Geometry: final body of the model. Coordinates: model frame, mm. Give positions to 0.01 mm unless a question says otherwise; leave off trailing zeros. Order: outer loops, then holes, each group sorted by start corner. A loop starts at its lowest first (then second) coordinate and runs counter-clockwise, first axis right, second up. Notation, with made-up numbers: M -18,19.5 L 21,19.5 A21 ccw 21,36.5 Z; hole C -39.75,86 d11. An arc over 180 degrees is marked long. Write item = value, one per line. Start each with the question number.
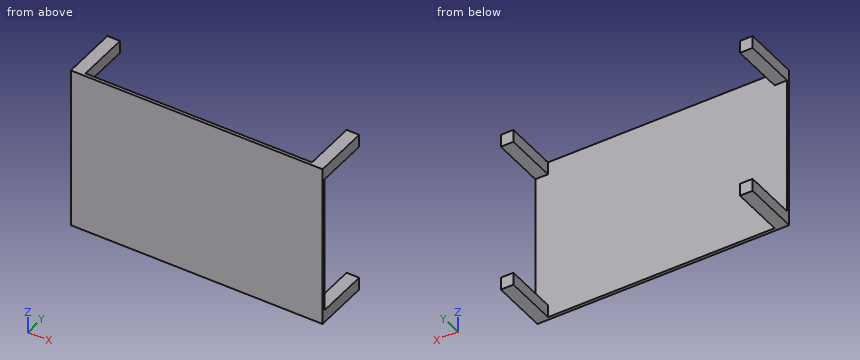
from build123d import *

# Parameters (mm, degrees)
SKETCH2_W            = 254
SKETCH2_H            = 165.1
BOSS_EXTRUDE1_DEPTH  = 3.175
SKETCH3_W            = 12.7
SKETCH3_H            = 12.7
BOSS_EXTRUDE2_DEPTH  = 53.975
LPATTERN1_COUNT      = 2
LPATTERN1_PITCH      = 152.4
LPATTERN1_COUNT_DIR2 = 2
LPATTERN1_PITCH_DIR2 = 241.3


with BuildPart() as part:
    # Sketch2 → Boss-Extrude1 (new body)
    with BuildSketch(Plane(origin=(0, 0, 0), x_dir=(1, 0, 0), z_dir=(0, 1, 0))):
        Rectangle(SKETCH2_W, SKETCH2_H)
    extrude(amount=BOSS_EXTRUDE1_DEPTH)

    # Sketch3 → Boss-Extrude2 (add)
    with BuildSketch(Plane(origin=(0, 3.175, 0), x_dir=(1, 0, 0), z_dir=(0, 1, 0))):
        with Locations((-120.65, -76.2)):
            Rectangle(SKETCH3_W, SKETCH3_H)
    boss_extrude2 = extrude(amount=BOSS_EXTRUDE2_DEPTH)

    # LPattern1: Boss-Extrude2 2 × 2
    with Locations(*[(j * LPATTERN1_PITCH_DIR2, 0, -i * LPATTERN1_PITCH) for i in range(LPATTERN1_COUNT) for j in range(LPATTERN1_COUNT_DIR2) if (i, j) != (0, 0)]):
        add(boss_extrude2)


solid = part.part
1) Cut plane C-C (z = -1). Return loops of the section in (x, y) (3 decimals), plus the area to 3 significant figures.
2) Cut plane A-A (y = 50.5). Return loops of the section in (x, z), plus the area to 3 significant figures.
3) Ray query, L1, parallel to X at y = 38, z = -70.5; L2, parallel to Y at x = 105, z = -28.5 (3 decimals). Return the intervals inside material, ascending.
4) Pin query (flat end, axial travel): pin 1 Ø1.5 at (x, z) = (-89, -38) entering from -Y. Return the tip coordinate at first contact, or that it passes through.
5) Cut plane B-B (x = 30). Return loops of the section in (y, z) (3 decimals), plus the area to 3 significant figures.
Reply:
q1.outline = M -127,0 L 127,0 L 127,3.175 L -127,3.175 Z
q1.area = 806 mm²
q2.outline = M -127,-82.55 L -114.3,-82.55 L -114.3,-69.85 L -127,-69.85 Z; M -127,69.85 L -114.3,69.85 L -114.3,82.55 L -127,82.55 Z; M 114.3,-82.55 L 127,-82.55 L 127,-69.85 L 114.3,-69.85 Z; M 114.3,69.85 L 127,69.85 L 127,82.55 L 114.3,82.55 Z
q2.area = 645 mm²
q3.L1 = -127 to -114.3, 114.3 to 127
q3.L2 = 0 to 3.175
q4.pin_1 = 0
q5.outline = M 0,-82.55 L 3.175,-82.55 L 3.175,82.55 L 0,82.55 Z
q5.area = 524 mm²
